Solid Edge part; units mm, degrees
sketch "Sketch1" plane through (0, 0, 0) normal (0, -1, 0) x (1, 0, 0)
  line L0 (0, 0) -> (2.8, 0)
  line L1 (2.8, 0) -> (1.5, -1.3)
  line L2 (1.5, -1.3) -> (1.5, -11.3)
  line L3 (1.5, -11.3) -> (0, -11.3)
  dimension "D1" = 1.5
revolve "RevolvedProtrusion1" add sketch "Sketch1" angle 360 about axis through (0, 0, -21.75) along (0, 0, 1)
chamfer "mounting_chamfer" distance 0.5 angle 45 1 edges at (-1.5, 0, -11.3)
sketch "Sketch2" plane through (0, 0, 0) normal (0, 0, 1) x (0, 1, 0)
  line L0 (0.5, -0.5) -> (1.5, -0.5)
  line L1 (1.5, -0.5) -> (1.5, 0.5)
  line L2 (1.5, 0.5) -> (0.5, 0.5)
  line L3 (0.5, 1.5) -> (0.5, 0.5)
  line L4 (-0.5, 1.5) -> (0.5, 1.5)
  line L5 (-0.5, 0.5) -> (-0.5, 1.5)
  line L6 (-0.5, 0.5) -> (-1.5, 0.5)
  line L7 (-1.5, 0.5) -> (-1.5, -0.5)
  line L8 (-1.5, -0.5) -> (-0.5, -0.5)
  line L9 (-0.5, -1.5) -> (-0.5, -0.5)
  line L10 (0.5, -1.5) -> (-0.5, -1.5)
  line L11 (0.5, -0.5) -> (0.5, -1.5)
  dimension "D1" = 0.5
extrude "plus_cutout" cut sketch "Sketch2" against normal blind 1.2
cosmetic_thread "Thread1"
properties part number "STD-DIN965-M3x15" material "Stainless steel"
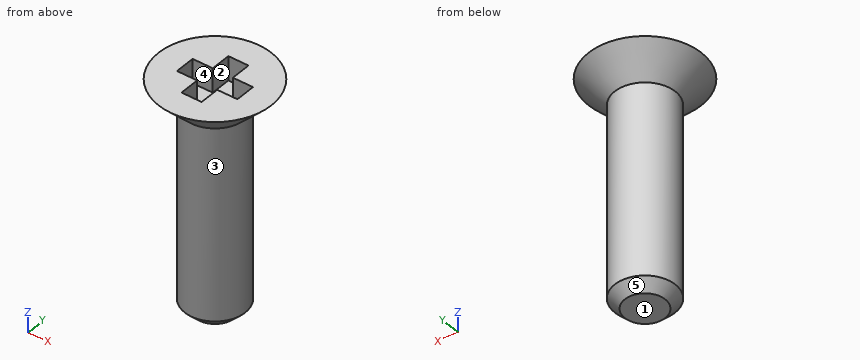
Input: part model. Units: mm. Frame: model coordinates. Face numbers are marked on the shaded views. A direction names the side the tool comes from. Coordinates: 2 decimals unless noted, no trailing zeros. Write each loop counter-clockwise with the first axis right and the second up, starting at its lowest first coordinate (ties: lowest second). Pieces come first, ordered by that corner, then holes. Notation, with made-up numbers: M -15,-38 L 0,-38 A24 cw 0,0 Z; hole C -18.5,23.5 d6. An arc over 180 degrees is marked long. Answer as a JSON object with one key per item and string values. Group by question number.
(1) Contact query for flat-ended pins moving along their axis: P1, Ø3, axis at x = -0.5, z = -3.5, coming from the +Y side; P2, Ø3, axis at x = 0, y = -1.5, coming from the +Z side; P3, Ø0.8, axis at x = 0, z = -0.5, coming from the +Y side; P4, Ø0.8, axis at x = 0, z = -0.5, coming from the -Y side. Output: stop coordinate, or through.
(2) Ray query, line 1 along Z through (x, y) = (-0.25, -0.25); line 2 along Y through (x, z) = (1.15, -5.75); line 3 along X through (y, z) = (0.45, -7). Return the intervals inside material, ascending. Write a range as [from, to].
(3) Set-up query: the marked faces 4 and 5. Return all of +Z, -Z, +X, -X, +Y, -Y with unobstructed straight access to the full face (end or side cutting, diameter ignored); none if empty.
(4) Section C-C on z = -5. Output: boundary loops of the cut face in (x, y), plus the area to 3 significant figures.
(5) Section A-A on x = 0. Output: boundary loops of the cut face in (y, z), plus the area to 3 significant figures.
(6) Mould query, pull axis X, two halves, no side actions, for the marked faces 1, 2 and 3. Classes: pulls with the +X half, pulls with the -X half, needs draft (parallel to the pull), parting line crosses it, or undercut.
Result set:
{
 "1": {"P1": "stops at y = 1.5", "P2": "stops at z = 0", "P3": "stops at y = 2.7", "P4": "stops at y = -2.7"},
 "2": {"line 1": "z = [-11.3, -1.2]", "line 2": "y = [-0.96, 0.96]", "line 3": "x = [-1.43, 1.43]"},
 "3": {"face 4": "+Z", "face 5": "-Z"},
 "4": {"outline": "C 0,0 d3", "area": "7.07 mm2"},
 "5": {"outline": "M -2.8,0 L -1.5,-1.3 L -1.5,-10.8 L -1,-11.3 L 1,-11.3 L 1.5,-10.8 L 1.5,-1.3 L 2.8,0 L 1.5,0 L 1.5,-1.2 L -1.5,-1.2 L -1.5,0 Z", "area": "31.7 mm2"},
 "6": {"face 1": "needs draft", "face 2": "undercut", "face 3": "parting line crosses it"}
}
